```python
from build123d import *
from build123d.topology import SkipClean

# Parameters (mm, degrees)
SKETCH_1_W                     = 22.22
SKETCH_1_H                     = 12.22
SKETCH_1_W_2                   = 15.22
SKETCH_1_H_2                   = 5.22
EXTRUDE_1_DEPTH                = 25
EXTRUDE_START                  = -2
SKETCH_3_W                     = 15.22
SKETCH_3_H                     = 5.22
EXTRUDE_2_DEPTH                = 9
SKETCH_4_W                     = 54.706051552
SKETCH_4_H                     = 5.2
CUT_EXTRUDE_1_DEPTH            = 5
SKETCH_5_W                     = 55.616807128
SKETCH_5_H                     = 5.2
CUT_EXTRUDE_2_DEPTH            = 5
FILLET_1_R                     = 2
PATTERN_LINEAR_1_COUNT         = 2
PATTERN_LINEAR_1_PITCH         = 10
FILLET_1_OF_PATTERN_LINEAR_1_R = 2
SKETCH_7_R                     = 1.65
CUT_EXTRUDE_5_DEPTH            = 29
CUT_EXTRUDE_START              = 1
CUT_EXTRUDE_7_OUTLINE_R        = 1.65
CUT_EXTRUDE_7_DEPTH            = 9
SKETCH_9_W                     = 15.22
SKETCH_9_H                     = 5.22
EXTRUDE_3_DEPTH                = 15
CUT_EXTRUDE_8_DEPTH            = 18
FILLET_2_R                     = 5
SKETCH_12_R                    = 1.6
CUT_EXTRUDE_9_DEPTH            = 16
SKETCH_13_R                    = 1.65
EXTRUDE_4_DEPTH                = 0.5
CUT_EXTRUDE_START_2            = -2.6
CUT_EXTRUDE_10_DEPTH           = 2.6
SKETCH_15_W                    = 15.22
SKETCH_15_H                    = 5.22
CUT_EXTRUDE_11_DEPTH           = 25.977155973
SKETCH_16_W                    = 15.22
SKETCH_16_H                    = 5.22
EXTRUDE_5_DEPTH                = 15
SKETCH_17_R                    = 1.6
CUT_EXTRUDE_12_DEPTH           = 34.48125775


# Read off the part's stored shape, not the designer's step: 切除-拉伸7
with BuildPart() as part:
    # 草图1 → 凸台-拉伸1 (new body)
    with BuildSketch(Plane(origin=(0, 0, 0), x_dir=(1, 0, 0), z_dir=(0, 1, 0))):
        Rectangle(SKETCH_1_W, SKETCH_1_H)
        Rectangle(SKETCH_1_W_2, SKETCH_1_H_2, mode=Mode.SUBTRACT)
    extrude(amount=EXTRUDE_1_DEPTH)

    # 草图3 → 凸台-拉伸2 (add)
    with BuildSketch(Plane(origin=(0, 12.5, 0), x_dir=(1, 0, 0), z_dir=(0, 1, 0)).offset(EXTRUDE_START)):
        Polygon((11.11, 0), (21.11, -11.11), (-21.11, -11.11), (-11.11, 0), (-21.11, 11.11), (21.11, 11.11), align=None)
        Rectangle(SKETCH_3_W, SKETCH_3_H, mode=Mode.SUBTRACT)
    extrude_2 = extrude(amount=EXTRUDE_2_DEPTH)

    # 草图4 → 切除-拉伸1 (cut)
    with BuildSketch(Plane(origin=(0, 0, -11.11), x_dir=(-1, 0, 0), z_dir=(0, 0, -1))):
        with Locations((0, 15)):
            Rectangle(SKETCH_4_W, SKETCH_4_H)
    cut_extrude_1 = extrude(amount=-CUT_EXTRUDE_1_DEPTH, mode=Mode.SUBTRACT)

    # 草图5 → 切除-拉伸2 (cut)
    with BuildSketch(Plane.XY.offset(11.11)):
        with Locations((0, 15)):
            Rectangle(SKETCH_5_W, SKETCH_5_H)
    cut_extrude_2 = extrude(amount=-CUT_EXTRUDE_2_DEPTH, mode=Mode.SUBTRACT)

    # 圆角1
    fillet_1_edges = [part.edges().sort_by_distance(p)[0] for p in [
        (-21.11, 18.55, 11.11),
        (21.11, 18.55, 11.11),
        (21.11, 11.45, 11.11),
        (-21.11, 11.45, 11.11),
        (-21.11, 11.45, -11.11),
        (21.11, 11.45, -11.11),
        (21.11, 18.55, -11.11),
        (-21.11, 18.55, -11.11),
    ]]
    fillet(fillet_1_edges, radius=FILLET_1_R)

    # 阵列(线性)1: 凸台-拉伸2, 切除-拉伸1, 切除-拉伸2 ×2
    with Locations(*[(0, -i * PATTERN_LINEAR_1_PITCH, 0) for i in range(1, PATTERN_LINEAR_1_COUNT)]):
        add(extrude_2)
        add(cut_extrude_1, mode=Mode.SUBTRACT)
        add(cut_extrude_2, mode=Mode.SUBTRACT)

    # 圆角1 of 阵列(线性)1
    fillet_1_of_pattern_linear_1_edges = [part.edges().sort_by_distance(p)[0] for p in [
        (-21.11, 8.55, 11.11),
        (21.11, 8.55, 11.11),
        (21.11, 1.45, 11.11),
        (-21.11, 1.45, 11.11),
        (-21.11, 1.45, -11.11),
        (21.11, 1.45, -11.11),
        (21.11, 8.55, -11.11),
        (-21.11, 8.55, -11.11),
    ]]
    fillet(fillet_1_of_pattern_linear_1_edges, radius=FILLET_1_OF_PATTERN_LINEAR_1_R)

    # 草图7 → 切除-拉伸5 (cut)
    with BuildSketch(Plane(origin=(0, 19.5, 0), x_dir=(1, 0, 0), z_dir=(0, 1, 0))):
        with Locations(Location((-10, 8.5, 0), (0, 0, 270))):
            Circle(SKETCH_7_R)
        with Locations(Location((10, 8.5, 0), (0, 0, 270))):
            Circle(SKETCH_7_R)
        with Locations(Location((10, -8.5, 0), (0, 0, 270))):
            Circle(SKETCH_7_R)
        with Locations(Location((-10, -8.5, 0), (0, 0, 270))):
            Circle(SKETCH_7_R)
    extrude(amount=-CUT_EXTRUDE_5_DEPTH, mode=Mode.SUBTRACT)

    # 切除-拉伸7 outline → 切除-拉伸7 (cut)
    # profile 1 of 2: a face of its own
    with BuildSketch(Plane(origin=(0, 9.5, 0), x_dir=(1, 0, 0), z_dir=(0, 1, 0)).offset(CUT_EXTRUDE_START)):
        with BuildLine():
            Line((-18.105496504, 7.771996616), (-11.11, 0))
            Line((-11.11, 0), (-11.11, 6.11))
            Line((-11.11, 6.11), (11.11, 6.11))
            Line((11.11, 6.11), (11.11, 0))
            Line((11.11, 0), (18.105496504, 7.771996616))
            ThreePointArc((18.105496504, 7.771996616), (18.4459951, 9.923631744), (16.618974744, 11.11))
            Line((16.618974744, 11.11), (-16.618974744, 11.11))
            ThreePointArc((-16.618974744, 11.11), (-18.4459951, 9.923631744), (-18.105496504, 7.771996616))
        make_face()
        with Locations((-10, 8.5)):
            Circle(CUT_EXTRUDE_7_OUTLINE_R, mode=Mode.SUBTRACT)
        with Locations((10, 8.5)):
            Circle(CUT_EXTRUDE_7_OUTLINE_R, mode=Mode.SUBTRACT)
    # profile 2 of 2: a face of its own
    with BuildSketch(Plane(origin=(0, 9.5, 0), x_dir=(1, 0, 0), z_dir=(0, 1, 0)).offset(CUT_EXTRUDE_START)):
        with BuildLine():
            Line((-11.11, -6.11), (-11.11, 0))
            Line((-11.11, 0), (-18.105496504, -7.771996616))
            ThreePointArc((-18.105496504, -7.771996616), (-18.4459951, -9.923631744), (-16.618974744, -11.11))
            Line((-16.618974744, -11.11), (16.618974744, -11.11))
            ThreePointArc((16.618974744, -11.11), (18.4459951, -9.923631744), (18.105496504, -7.771996616))
            Line((18.105496504, -7.771996616), (11.11, 0))
            Line((11.11, 0), (11.11, -6.11))
            Line((11.11, -6.11), (-11.11, -6.11))
        make_face()
        with Locations((10, -8.5)):
            Circle(CUT_EXTRUDE_7_OUTLINE_R, mode=Mode.SUBTRACT)
        with Locations((-10, -8.5)):
            Circle(CUT_EXTRUDE_7_OUTLINE_R, mode=Mode.SUBTRACT)
    extrude(amount=CUT_EXTRUDE_7_DEPTH, mode=Mode.SUBTRACT)

    # 草图9 → 凸台-拉伸3 (add)
    with BuildSketch(Plane.XZ):
        Rectangle(SKETCH_9_W, SKETCH_9_H)
    extrude(amount=-EXTRUDE_3_DEPTH)

    # 草图11 → 切除-拉伸8 (cut)
    with BuildSketch(Plane(origin=(0, 9.5, 0), x_dir=(1, 0, 0), z_dir=(0, 1, 0))):
        with BuildLine():
            Line((11.11, 0), (18.105496504, 7.771996616))
            ThreePointArc((18.105496504, 7.771996616), (18.4459951, 9.923631744), (16.618974744, 11.11))
            Line((16.618974744, 11.11), (-16.618974744, 11.11))
            ThreePointArc((-16.618974744, 11.11), (-18.4459951, 9.923631744), (-18.105496504, 7.771996616))
            Line((-18.105496504, 7.771996616), (-11.11, 0))
            Line((-11.11, 0), (-11.11, 6.11))
            Line((-11.11, 6.11), (11.11, 6.11))
            Line((11.11, 6.11), (11.11, 0))
        make_face()
    extrude(amount=-CUT_EXTRUDE_8_DEPTH, mode=Mode.SUBTRACT)

    # 圆角2
    fillet_2_edges = [part.edges().sort_by_distance(p)[0] for p in [
        (11.11, 12.5, -6.11),
        (11.11, 17.25, 6.11),
        (-11.11, 17.25, 6.11),
        (-11.11, 12.5, -6.11),
    ]]
    fillet(fillet_2_edges, radius=FILLET_2_R)

    # 草图12 → 切除-拉伸9 (cut)
    with BuildSketch(Plane(origin=(0, 0, -6.11), x_dir=(-1, 0, 0), z_dir=(0, 0, -1))):
        with Locations((-4, 18.5)):
            Circle(SKETCH_12_R)
        with Locations((4, 18.5)):
            Circle(SKETCH_12_R)
        with Locations((-4, 12.5)):
            Circle(SKETCH_12_R)
        with Locations((4, 12.5)):
            Circle(SKETCH_12_R)
    extrude(amount=-CUT_EXTRUDE_9_DEPTH, mode=Mode.SUBTRACT)

    # 草图13 → 凸台-拉伸4 (add)
    with SkipClean():  # the faces are left unmerged after this step: merging them gives an invalid solid
        with BuildSketch(Plane.XZ.offset(-0.5)):
            with BuildLine():
                Line((11.11, 0), (18.105496504, 7.771996616))
                ThreePointArc((18.105496504, 7.771996616), (18.4459951, 9.923631744), (16.618974744, 11.11))
                Line((16.618974744, 11.11), (-16.618974744, 11.11))
                ThreePointArc((-16.618974744, 11.11), (-18.4459951, 9.923631744), (-18.105496504, 7.771996616))
                Line((-18.105496504, 7.771996616), (-11.11, 0))
                Line((-11.11, 0), (-11.11, 6.11))
                Line((-11.11, 6.11), (11.11, 6.11))
                Line((11.11, 6.11), (11.11, 0))
            make_face()
            with Locations(Location((-10, 8.5, 0), (0, 0, 270))):
                Circle(SKETCH_13_R, mode=Mode.SUBTRACT)
            with Locations(Location((10, 8.5, 0), (0, 0, 270))):
                Circle(SKETCH_13_R, mode=Mode.SUBTRACT)
        extrude(amount=EXTRUDE_4_DEPTH)

    # 草图14 → 切除-拉伸10 (cut)
    with BuildSketch(Plane.XZ.offset(CUT_EXTRUDE_START_2)):
        with BuildLine():
            Line((-6.11, -6.11), (6.11, -6.11))
            ThreePointArc((6.11, -6.11), (9.645533906, -4.645533906), (11.11, -1.11))
            Line((11.11, -1.11), (11.11, 0))
            Line((11.11, 0), (18.105496504, 7.771996616))
            ThreePointArc((18.105496504, 7.771996616), (18.4459951, 9.923631744), (16.618974744, 11.11))
            Line((16.618974744, 11.11), (-16.618974744, 11.11))
            ThreePointArc((-16.618974744, 11.11), (-18.4459951, 9.923631744), (-18.105496504, 7.771996616))
            Line((-18.105496504, 7.771996616), (-11.11, 0))
            Line((-11.11, 0), (-11.11, -1.11))
            ThreePointArc((-11.11, -1.11), (-9.645533906, -4.645533906), (-6.11, -6.11))
        make_face()
    extrude(amount=CUT_EXTRUDE_10_DEPTH, mode=Mode.SUBTRACT)

    # 草图15 → 切除-拉伸11 (cut, through all)
    with BuildSketch(Plane(origin=(0, 15, 0), x_dir=(1, 0, 0), z_dir=(0, 1, 0))):
        Rectangle(SKETCH_15_W, SKETCH_15_H)
    extrude(amount=-CUT_EXTRUDE_11_DEPTH, mode=Mode.SUBTRACT)

    # 草图16 → 凸台-拉伸5 (add)
    with BuildSketch(Plane.XZ.offset(-2.6)):
        with BuildLine():
            Line((11.11, -1.11), (11.11, 1.11))
            ThreePointArc((11.11, 1.11), (9.645533906, 4.645533906), (6.11, 6.11))
            Line((6.11, 6.11), (-6.11, 6.11))
            ThreePointArc((-6.11, 6.11), (-9.645533906, 4.645533906), (-11.11, 1.11))
            Line((-11.11, 1.11), (-11.11, -1.11))
            ThreePointArc((-11.11, -1.11), (-9.645533906, -4.645533906), (-6.11, -6.11))
            Line((-6.11, -6.11), (6.11, -6.11))
            ThreePointArc((6.11, -6.11), (9.645533906, -4.645533906), (11.11, -1.11))
        make_face()
        Rectangle(SKETCH_16_W, SKETCH_16_H, mode=Mode.SUBTRACT)
    extrude(amount=EXTRUDE_5_DEPTH)

    # 草图17 → 切除-拉伸12 (cut, through all)
    with BuildSketch(Plane.XY.offset(6.11)):
        with Locations(Location((-4, 12.5, 0), (0, 0, 180))):
            Circle(SKETCH_17_R)
        with Locations(Location((4, 12.5, 0), (0, 0, 180))):
            Circle(SKETCH_17_R)
        with Locations((-4, -9.5)):
            Circle(SKETCH_17_R)
        with Locations((4, -9.5)):
            Circle(SKETCH_17_R)
        with Locations((-4, -4.5)):
            Circle(SKETCH_17_R)
        with Locations((4, -4.5)):
            Circle(SKETCH_17_R)
        with Locations((-4, 0.5)):
            Circle(SKETCH_17_R)
        with Locations((4, 0.5)):
            Circle(SKETCH_17_R)
    extrude(amount=-CUT_EXTRUDE_12_DEPTH, mode=Mode.SUBTRACT)


solid = part.part
```
Check sheet for the modelled part. Datum: model origin and axes. Units: mm. A direction names the side the tool comes from. Give positions to 0.01 mm unless a question says otherwise; leave off trailing zeros. Loops run counter-clockwise (first coordinate to the right, second up) from the corner with the lowest first, then second, coordinate; pieces in that order, holes last. Notation, with made-up numbers: M 10,-30 L 65,-30 A7 cw 65,-18 Z; hole C -26,67.25 d1. An arc over 180 degrees is marked long. Answer in a Markdown table with one row per item.
1) Cross-section at A-A (y = 12.5). Enter the section's corners in (x, z), plus the area to 3 significant figures.
Solutions:
| item | result |
|---|---|
| outline | M -11.11,-1.11 A5 ccw -6.11,-6.11 L -5.6,-6.11 L -5.6,-2.61 L -7.61,-2.61 L -7.61,2.61 L -5.6,2.61 L -5.6,6.11 L -6.11,6.11 A5 ccw -11.11,1.11 Z; M -2.4,-6.11 L 2.4,-6.11 L 2.4,-2.61 L -2.4,-2.61 Z; M -2.4,2.61 L 2.4,2.61 L 2.4,6.11 L -2.4,6.11 Z; M 5.6,-6.11 L 6.11,-6.11 A5 ccw 11.11,-1.11 L 11.11,1.11 A5 ccw 6.11,6.11 L 5.6,6.11 L 5.6,2.61 L 7.61,2.61 L 7.61,-2.61 L 5.6,-2.61 Z |
| area | 126 mm^2 |
2) Cross-section at B-B (x = -10). Enter the section's corners in (y, z), plus the area to 3 significant figures.
Solutions:
| item | result |
|---|---|
| outline | M -12.4,-4.25 L 25,-4.25 L 25,4.25 L 9.5,4.25 L 9.5,6.85 L 7.6,6.85 L 7.6,6.11 L 2.6,6.11 L 2.6,4.25 L -12.4,4.25 Z; M 7.6,10.15 L 9.5,10.15 L 9.5,11.11 L 7.6,11.11 Z |
| area | 334 mm^2 |
3) Depth check by flat-ended pin: pin 1 (10 mm diameter, centred on x = -2, y = 15, fed in from +Z); pin 2 (3 mm diameter, centred on x = -8.5, y = 19.5, fed in from +Z); pin 3 (5 mm diameter, centred on x = -4, y = 12.5, fed in from -Z); pin 4 (2.5 mm diameter, centred on y = 12.5, z = -1, fed in from +X). Enter the tip coordinate at first touch or a pass-through.
Solutions:
| item | result |
|---|---|
| pin 1 | stops at z = 6.11 |
| pin 2 | stops at z = 6.03 |
| pin 3 | stops at z = -6.11 |
| pin 4 | stops at x = 11.11 |
4) Tool access check on faces 5 (the face through (5.18, 13.58, 4.34)), 6 (the face through (9.68, -4.8, 4.61)), 7 (the face through (0, 0, 6.11)), 8 (the face through (9.61, 17.36, 4.68)), 9 (the face through (-7.61, 7, 0)). Record the directions out of +Z, -Z, +X, -X, +Y, -Y that give a thin tool (end or side, any length) a straight path to the whole face; none if there is none.
Solutions:
| item | result |
|---|---|
| face 5 | +Z, -Z |
| face 6 | +Z, +X, -Y |
| face 7 | +Z, +X, -X, -Y |
| face 8 | +Z, +X, +Y |
| face 9 | +Y, -Y |
5) Mould release check, pull along Z, two halves, no side actions. Record for faces 1 (the face through (-9.61, -4.8, 4.68)), 2 (the face through (7.61, 7, 0)), 3 (the face through (-5.6, 0.57, -4.34)), 4 (the face through (0, 7, 2.61)): released by +Z, released by -Z, zero draft, split by the parting line, or undercut.
Solutions:
| item | result |
|---|---|
| face 1 | released by +Z |
| face 2 | undercut |
| face 3 | zero draft |
| face 4 | undercut |
6) Thickness scan on line 1 (Y direction, x = -4, z = -5.1); line 2 (X direction, y = 9.15, z = 8.5); line 3 (Z direction, x = 6.5, y = 8). Record the ranges inside material, lowest first.
Solutions:
| item | result |
|---|---|
| line 1 | y = -12.4 to -11.1, -7.9 to -6.1, -2.9 to -1.1, 2.1 to 10.9, 14.1 to 16.9, 20.1 to 25 |
| line 2 | x = -18.52 to -11.65, -8.35 to 8.35, 11.65 to 18.52 |
| line 3 | z = -6.09 to -2.61, 2.61 to 11.11 |
7) Cross-section at C-C (z = -3.25). Count the separate pieces of the cut face and the enclosed holes in it, plus the area to 3 significant figures.
Solutions:
| item | result |
|---|---|
| separate pieces | 1 |
| enclosed holes | 10 |
| area | 715 mm^2 |
